For this review, take the finished solid that the model builds, in its own axes (mm). Face numbers are marked on the shaded views. A direction names the side the tool comes from. Give positions to 0.01 mm unless a question says otherwise; leave off trailing zeros. Write each loop counter-clockwise with the first axis right and the second up, starting at its lowest first coordinate (ties: lowest second). Pieces come first, ordered by that corner, then holes. Notation, with made-up numbers: (80, 29) -> (117, 29) arc R14 cw to (117, 45) -> close; hole circle Ø10 at (80, 53). An arc over 180 degrees is marked (long way). Write item = value, one per line.
```python
from build123d import *

# Parameters (mm, degrees)
EXTRUDE_1_DEPTH     = 30
EXTRUDE_2_DEPTH     = 6
CUT_EXTRUDE_1_DEPTH = 6
CUT_EXTRUDE_2_DEPTH = 6
FILLET_1_R          = 10
FILLET_2_R          = 3


with BuildPart() as part:
    # 草图1 → 凸台-拉伸1 (new body)
    with BuildSketch(Plane(origin=(0, 0, 0), x_dir=(0, 0, -1), z_dir=(1, 0, 0))):
        Polygon((0, 0), (25, 0), (25, 2), (2, 2), (2, 17), (0, 17), align=None)
    extrude(amount=EXTRUDE_1_DEPTH)

    # 草图3 → 凸台-拉伸2 (add)
    with BuildSketch(Plane(origin=(0, 17, 0), x_dir=(1, 0, 0), z_dir=(0, 1, 0))):
        Polygon((0, 0), (0, -7), (7, -7), (7, -5), (2, -5), (2, 0), align=None)
        Polygon((28, -5), (28, 0), (30, 0), (30, -7), (23, -7), (23, -5), align=None)
    extrude(amount=-EXTRUDE_2_DEPTH)

    # 草图4 → 切除-拉伸1 (cut)
    with BuildSketch(Plane.XY.offset(7)):
        with BuildLine():
            Line((22.34696537, 14.9), (27, 14.9))
            ThreePointArc((27, 14.9), (27.9, 14), (27, 13.1))
            Line((27, 13.1), (22.34696537, 13.1))
            ThreePointArc((22.34696537, 13.1), (21.44696537, 14), (22.34696537, 14.9))
        make_face()
        with BuildLine():
            Line((7.65303463, 14.9), (3, 14.9))
            ThreePointArc((3, 14.9), (2.1, 14), (3, 13.1))
            Line((3, 13.1), (7.65303463, 13.1))
            ThreePointArc((7.65303463, 13.1), (8.55303463, 14), (7.65303463, 14.9))
        make_face()
    extrude(amount=-CUT_EXTRUDE_1_DEPTH, mode=Mode.SUBTRACT)

    # 草图5 → 切除-拉伸2 (cut)
    with BuildSketch(Plane(origin=(0, 2, 0), x_dir=(1, 0, 0), z_dir=(0, 1, 0))):
        with BuildLine():
            Line((16.05, 25.529105391), (16.05, 11.529105391))
            ThreePointArc((16.05, 11.529105391), (15, 10.479105391), (13.95, 11.529105391))
            Line((13.95, 11.529105391), (13.95, 25.529105391))
            ThreePointArc((13.95, 25.529105391), (15, 26.579105391), (16.05, 25.529105391))
        make_face()
    extrude(amount=-CUT_EXTRUDE_2_DEPTH, mode=Mode.SUBTRACT)

    # 圆角1
    fillet_1_edges = [part.edges().sort_by_distance(p)[0] for p in [
        (30, 1, -25),
        (0, 1, -25),
    ]]
    fillet(fillet_1_edges, radius=FILLET_1_R)

    # 圆角2
    # the kernel refuses this fillet: 3 mm, written as the material it takes off along each edge
    with BuildSketch(Plane(origin=(30, 17, -9.5), x_dir=(0, -1, 0), z_dir=(0, 0, 1)), Plane(origin=(0, 17, 14.5), x_dir=(0, -1, 0), z_dir=(0, 0, -1))) as fillet_2_piece_1:
        with BuildLine():
            CenterArc((FILLET_2_R, -FILLET_2_R), FILLET_2_R, 90, 90)
            Line((0, -FILLET_2_R), (0, 0))
            Line((0, 0), (FILLET_2_R, 0))
        make_face()
    extrude(amount=24, mode=Mode.SUBTRACT)


solid = part.part
```
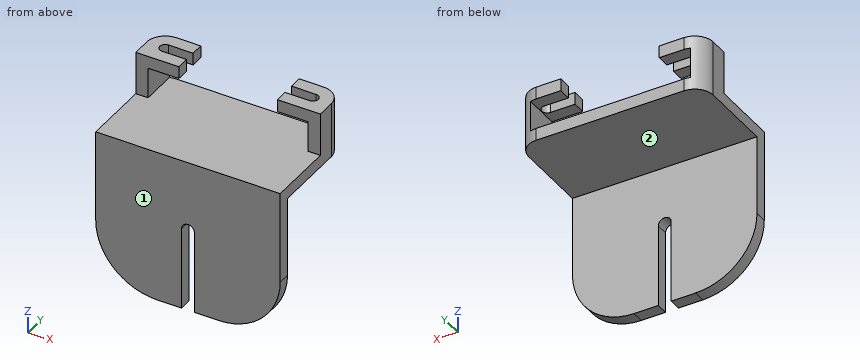
(1) Take a section at B-B (y = 1.25). Write out the cut boundary in (x, z), plus the area to 3 significant figures.
Answers below:
outline = (0, -15) arc R10 ccw to (10, -25) -> (13.95, -25) -> (13.95, -11.53) arc R1.05 cw to (16.05, -11.53) -> (16.05, -25) -> (20, -25) arc R10 ccw to (30, -15) -> (30, 0) -> (0, 0) -> close
area = 677 mm^2
(2) To check wall thickness, follow probe 1 along X at (y, z) = (13.25, 3); probe 2 along Y at (x, z) = (20.5, -17); probe 3 along Z at (x, y) = (22.75, 13.5). State the ranges of each line that lie inside material, in increasing order.
Answers below:
probe_1 = 0 to 2, 28 to 30
probe_2 = 0 to 2
probe_3 = -2 to 0
(3) For pin 1 (2 mm diameter, centred on x = 16.5, y = 9, fed in from -Z); pin 2 (3.5 mm diameter, centred on x = 5, z = 4, fed in from -Y); pin 3 (2 mm diameter, centred on x = 18.5, y = 8, fed in from +Z); pin 4 (10 mm diameter, centred on y = 11.5, z = -19.5, fed in from +X), all flat-tipped, find the tip position at first contact; note any pin that passes through.
Answers below:
pin_1 = -2
pin_2 = 11
pin_3 = 0
pin_4 = through
(4) Take a section at C-C (x = 15). Write out the cut boundary in (y, z).
Answers below:
outline = (0, -10.48) -> (2, -10.48) -> (2, -2) -> (17, -2) -> (17, 0) -> (0, 0) -> close
(5) Take a section at D-D (x = 9). Write out the cut boundary in (y, z).
Answers below:
outline = (0, -24.95) -> (2, -24.95) -> (2, -2) -> (17, -2) -> (17, 0) -> (0, 0) -> close
(6) Tool access review of the marked faces 1 and 2: name each direction out of +Z, -Z, +X, -X, +Y, -Y from which nothing blocks a thin tool from reaching the whole face with its end or side.
Answers below:
face_1 = +Z, -Z, +X, -X, -Y
face_2 = -Z, +X, -X, +Y
(7) Take a section at A-A (x = 3.5). Write out the cut boundary in (y, z), plus the area to 3 significant figures.
Answers below:
outline = (0, -22.6) -> (2, -22.6) -> (2, -2) -> (17, -2) -> (17, 0) -> (0, 0) -> close; (11, 5) -> (13.1, 5) -> (13.1, 7) -> (11, 7) -> close; (14.9, 5) -> (17, 5) -> (17, 7) -> (14.9, 7) -> close
area = 83.6 mm^2
